from build123d import *

# Parameters (mm, degrees)
SKETCH_4_R                       = 14
EXTRUDE_1_DEPTH                  = 10
EXTRUDE_2_DEPTH                  = 10
FILLET_1_R                       = 0.5
PATTERN_CIRCULAR_1_COUNT         = 8
FILLET_1_OF_PATTERN_CIRCULAR_1_R = 0.5
CUT_EXTRUDE_1_DEPTH              = 28.30524858


with BuildPart() as part:
    # Sketch 4 → Extrude 1 (new body)
    with BuildSketch(Plane(origin=(0, 0, 0), x_dir=(1, 0, 0), z_dir=(0, 1, 0))):
        with Locations(Location((0, 0, 0), (0, 0, 270))):
            Circle(SKETCH_4_R)
    extrude(amount=EXTRUDE_1_DEPTH)

    # Sketch 3 → Extrude 2 (add)
    with BuildSketch(Plane(origin=(0, 0, 0), x_dir=(1, 0, 0), z_dir=(0, 1, 0))):
        with BuildLine():
            Line((0.224080336, 15.033412012), (0.224080336, 13.9982066))
            ThreePointArc((0.224080336, 13.9982066), (-2.731264508, 13.730993926), (-5.563904985, 12.846904737))
            Line((-5.563904985, 12.846904737), (-5.960060945, 13.80330983))
            add(Edge.make_bspline(
                [(-5.858426114, 17.019954273), (-5.920939237, 16.775820636), (-6.005177259, 16.385669184), (-6.081389407, 15.859669081), (-6.117456435, 15.463573167), (-6.130866377, 15.108674888), (-6.126107546, 14.796141282), (-6.107718221, 14.526781883), (-6.080279115, 14.301036558), (-6.048330179, 14.119000945), (-6.01650055, 13.980359087), (-5.987708331, 13.879742422), (-5.969195203, 13.825538164), (-5.960060945, 13.80330983)],
                knots=[0, 0, 0, 0, 0.232146242, 0.367277189, 0.48933989, 0.598334347, 0.694260559, 0.777118527, 0.846908252, 0.903629737, 0.947282983, 0.977868, 1, 1, 1, 1], degree=3))
            ThreePointArc((-5.858426114, 17.019954273), (-3.511625796, 17.654135047), (-1.10077454, 17.966310011))
            add(Edge.make_bspline(
                [(-1.10077454, 17.966310011), (-0.949594047, 17.764682676), (-0.722463767, 17.436466231), (-0.450761398, 16.979670628), (-0.265860465, 16.627527975), (-0.117657603, 16.304776481), (-0.002452756, 16.014211953), (0.083637102, 15.758319028), (0.14467567, 15.539257051), (0.184820715, 15.358851746), (0.208469915, 15.218582699), (0.220373703, 15.114606716), (0.224012874, 15.057443845), (0.224080336, 15.033412012)],
                knots=[0, 0, 0, 0, 0.232146242, 0.367277189, 0.48933989, 0.598334347, 0.694260559, 0.777118527, 0.846908252, 0.903629737, 0.947282983, 0.977868, 1, 1, 1, 1], degree=3))
        make_face()
    extrude_2 = extrude(amount=EXTRUDE_2_DEPTH)

    # Fillet 1
    fillet_1_edges = [part.edges().sort_by_distance(p)[0] for p in [
        (-5.563904985, 5, -12.846904737),
        (0.224080336, 5, -13.9982066),
    ]]
    fillet(fillet_1_edges, radius=FILLET_1_R)

    # Pattern Circular 1: Extrude 2 ×8 about axis
    pattern_circular_1_axis = Axis((0, 10, 0), (0, 1, 0))
    for i in range(1, PATTERN_CIRCULAR_1_COUNT):
        add(extrude_2.rotate(pattern_circular_1_axis, i * 360 / PATTERN_CIRCULAR_1_COUNT))

    # Fillet 1 of Pattern Circular 1
    fillet_1_of_pattern_circular_1_edges = [part.edges().sort_by_distance(p)[0] for p in [
        (-13.018408401, 5, -5.149858512),
        (-9.739778086, 5, -10.056675536),
        (-12.846904737, 5, 5.563904985),
        (-13.9982066, 5, -0.224080336),
        (-5.149858512, 5, 13.018408401),
        (-10.056675536, 5, 9.739778086),
        (5.563904985, 5, 12.846904737),
        (-0.224080336, 5, 13.9982066),
        (13.018408401, 5, 5.149858512),
        (9.739778086, 5, 10.056675536),
        (12.846904737, 5, -5.563904985),
        (13.9982066, 5, 0.224080336),
        (5.149858512, 5, -13.018408401),
        (10.056675536, 5, -9.739778086),
    ]]
    fillet(fillet_1_of_pattern_circular_1_edges, radius=FILLET_1_OF_PATTERN_CIRCULAR_1_R)

    # Sketch 5 → Cut-Extrude 1 (cut, through all)
    with BuildSketch(Plane(origin=(0, 10, 0), x_dir=(1, 0, 0), z_dir=(0, 1, 0))):
        with BuildLine():
            Line((-1.148521284, 2.879392099), (-0.571628971, 2.764641083))
            Line((-0.571628971, 2.764641083), (0.228241349, 6.785860733))
            Line((0.228241349, 6.785860733), (2.385968966, 6.356662024))
            Line((2.385968966, 6.356662024), (1.586098646, 2.335442375))
            Line((1.586098646, 2.335442375), (2.162990959, 2.220691359))
            ThreePointArc((2.162990959, 2.220691359), (-0.604779998, -3.040434369), (-1.148521284, 2.879392099))
        make_face()
    extrude(amount=-CUT_EXTRUDE_1_DEPTH, mode=Mode.SUBTRACT)


solid = part.part
Check sheet for the modelled part. Datum: model origin and axes. Units: mm. A direction names the side the tool comes from. Give positions to 0.01 mm unless a question says otherwise; leave off trailing zeros. Answer as a JSON object with one key per item and string values. Group by question number.
Q1. Go/stop test with flat-tipped pins: P1, Ø5, axis at y = 4, z = -4.5, coming from the -X side; P2, Ø4, axis at y = 1.5, z = 10, coming from the -X side; P3, Ø3, axis at y = 4, z = -12, coming from the +X side. Record where each tip stops, or that it passes through.
Q2. Release check for a two-part mould opening along Z. For faces 6 (the cylindrical face through (-2.759, 4.93, 13.725)), 7 (the cylindrical face through (17.647, 4.93, -3.545)), 8 (the flat face through (-0.177, 5.07, -4.747)) record: released by +Z, released by -Z, zero draft, split by the parting line, or undercut.
Q3. Access from +Z, -Z, +X, -X, +Y, -Y to the whole of each face (thin tool, end or side, straight path). Record for faces 1 (the cylindrical face through (13.725, 4.93, 2.759)), 2 (the flat face through (1.292, 5.07, -6.574)), 3 (the flat face through (0, 0, 4)), 4 (the cylindrical face through (3.545, 4.93, 17.647)), 5 (the cylindrical face through (-13.725, 4.93, -2.759)).
Q4. Material ranges on line 1 along X through (y, z) = (2.25, 15); line 2 along X through (y, z) = (9, -11); line 3 along X through (y, z) = (2, 12.5), recorded low to high. Write a range as [from, to].
Evaluation:
{
 "1": {"P1": "stops at x = -15.58", "P2": "stops at x = -11.58", "P3": "stops at x = 11.93"},
 "2": {"face 6": "released by +Z", "face 7": "released by -Z", "face 8": "undercut"},
 "3": {"face 1": "+X, +Y, -Y", "face 2": "+Y, -Y", "face 3": "+Z, -Z, +X, -X, -Y", "face 4": "+Z, +X, +Y, -Y", "face 5": "-X, +Y, -Y"},
 "4": {"line 1": "x = [-9.95, -6.33], [-0.22, 6.13]", "line 2": "x = [-14.25, -10.75], [-8.66, 11.15]", "line 3": "x = [-11.73, 6.3]"}
}
